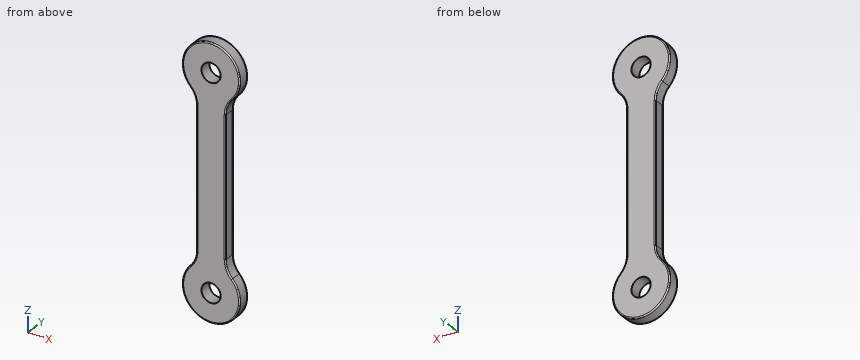
```python
from build123d import *

# Parameters (mm, degrees)
SKETCH1_R           = 2
BOSS_EXTRUDE1_DEPTH = 2.5
FILLET1_R           = 5
FILLET2_R           = 0.25


with BuildPart() as part:
    # Sketch1 → Boss-Extrude1 (new body)
    with BuildSketch(Plane(origin=(0, 0, 0), x_dir=(1, 0, 0), z_dir=(0, 1, 0))):
        with BuildLine():
            ThreePointArc((-3, -16.803847577), (0, -28), (3, -16.803847577))
            Line((3, -16.803847577), (3, 16.803847577))
            ThreePointArc((3, 16.803847577), (0, 28), (-3, 16.803847577))
            Line((-3, 16.803847577), (-3, -16.803847577))
        make_face()
        with Locations((0, -22)):
            Circle(SKETCH1_R, mode=Mode.SUBTRACT)
        with Locations((0, 22)):
            Circle(SKETCH1_R, mode=Mode.SUBTRACT)
    extrude(amount=BOSS_EXTRUDE1_DEPTH)

    # Fillet1
    fillet1_edges = [part.edges().sort_by_distance(p)[0] for p in [
        (-3, 1.25, 16.803847577),
        (-3, 1.25, -16.803847577),
        (3, 1.25, -16.803847577),
        (3, 1.25, 16.803847577),
    ]]
    fillet(fillet1_edges, radius=FILLET1_R)

    # Fillet2
    fillet2_edges = [part.edges().sort_by_distance(p)[0] for p in [
        (0, 0, -28),
        (0, 2.5, -28),
        (3, 0, 0),
        (3, 2.5, 0),
        (0, 0, 28),
        (0, 2.5, 28),
        (-3, 0, 0),
        (-3, 2.5, 0),
        (3.353398114, 0, -16.296537929),
        (3.353398114, 2.5, -16.296537929),
        (3.353398114, 0, 16.296537929),
        (3.353398114, 2.5, 16.296537929),
        (-3.353398114, 0, 16.296537929),
        (-3.353398114, 2.5, 16.296537929),
        (-3.353398114, 0, -16.296537929),
        (-3.353398114, 2.5, -16.296537929),
    ]]
    fillet(fillet2_edges, radius=FILLET2_R)


solid = part.part
```
Part model, mm, in its own coordinate system. Round coordinates to 2 decimals unless told otherwise and drop trailing zeros. Write each loop counter-clockwise with the first axis right and the second up, starting at its lowest first coordinate (ties: lowest second). Pieces come first, ordered by that corner, then holes.
Item 1: Drop flat-ended pins along their axis: pin 1 Ø0.6 at (y, z) = (1, 7) entering from -X; pin 2 Ø1 at (x, y) = (-4, 2) entering from +Z. Give the stop position or say it passes through.
Results:
pin 1: stops at x = -3
pin 2: stops at z = 26.87
Item 2: Cut at B-B, the plane y = 0.9. Give the cut face in (x, z).
Results:
outline: (-4.36, -17.88) arc R6 ccw (long way) to (4.36, -17.88) arc R5 cw to (3, -14.45) - (3, 14.45) arc R5 cw to (4.36, 17.88) arc R6 ccw (long way) to (-4.36, 17.88) arc R5 cw to (-3, 14.45) - (-3, -14.45) arc R5 cw to start; hole circle Ø4 at (0, -22); hole circle Ø4 at (0, 22)
Item 3: Cut at C-C, the plane z = -12. Give the cut face in (x, y), plus the area to 3 significant figures.
Results:
outline: (-3, 0.25) arc R0.25 ccw to (-2.75, 0) - (2.75, 0) arc R0.25 ccw to (3, 0.25) - (3, 2.25) arc R0.25 ccw to (2.75, 2.5) - (-2.75, 2.5) arc R0.25 ccw to (-3, 2.25) - close
area: 14.9 mm2
Item 4: Probe L1, parallel to Z at x = 0, y = 1.05; L2, parallel to X at y = 1.9, z = 22; L3, parallel to X at y = 0.7, z = -1. List the from-to ranges inside material, lowest first.
Results:
L1: z = -28 to -24, -20 to 20, 24 to 28
L2: x = -6 to -2, 2 to 6
L3: x = -3 to 3
Item 5: Cut at A-A, the plane x = 0. Give the cut face in (y, z).
Results:
outline: (0, -27.75) arc R0.25 ccw to (0.25, -28) - (2.25, -28) arc R0.25 ccw to (2.5, -27.75) - (2.5, -24) - (0, -24) - close; (0, -20) - (2.5, -20) - (2.5, 20) - (0, 20) - close; (0, 24) - (2.5, 24) - (2.5, 27.75) arc R0.25 ccw to (2.25, 28) - (0.25, 28) arc R0.25 ccw to (0, 27.75) - close
